Design review of the part shown in the three views and the two pictorial views. Dimensions are in mm from the part's minimum x, y and z. Coordinates: 2 decimals unless noted, no trailing zeros. Loops run counter-clockwise (first coordinate to the right, second up) from the corner with the lowest first, then second, coordinate; pieces in that order, holes last.
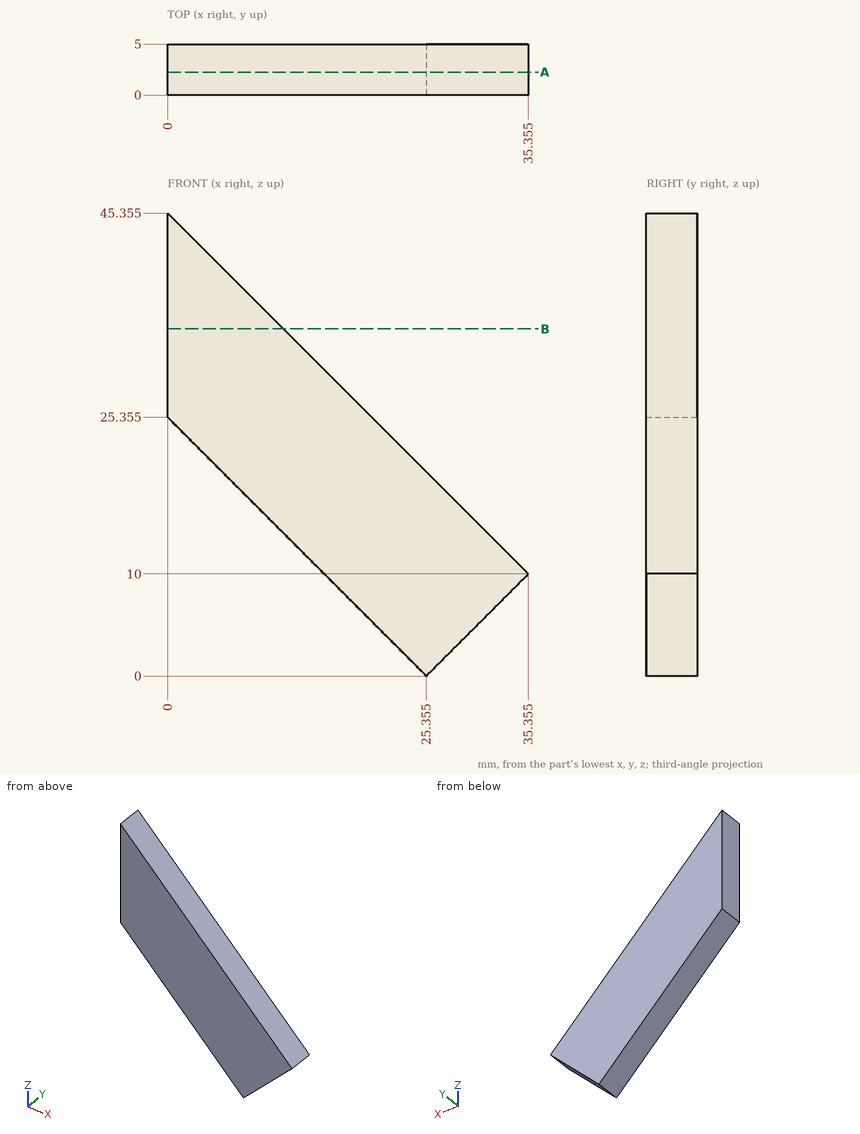
Q1. Consider section B-B (z = 34). State the section outline as (x, y) points (1 decimal), then the cut area to 3 significant figures.
Q2. For pin 1 Ø3 at (x, y) = (4.5, 3.5) entering from -Z (1 decimal), flat-tipped, find the tip position at first contact; note if it passes through.
Q3. Consider section A-A (y = 2.25). State the section outline as (x, z) points (1 decimal), then the cut area to 3 significant figures.
Q4. Wall thickness on probe 1 along Z at (x, y) = (30, 2.4) (1 decimal); probe 2 along Z at (x, y) = (4, 3.3) (1 decimal); probe 3 along X at (y, z) = (4.1, 33.5) (1 decimal): over which ranges is each line inside the solid? List them lowest first.
Model answer:
1. outline: (0, 0) - (11.4, 0) - (11.4, 5) - (0, 5) - close
1. area: 56.8 mm2
2. pin 1: stops at z = 19.4
3. outline: (0, 25.4) - (25.4, 0) - (35.4, 10) - (0, 45.4) - close
3. area: 607 mm2
4. probe 1: z = 4.6 to 15.4
4. probe 2: z = 21.4 to 41.4
4. probe 3: x = 0 to 11.9
